The listing builds one solid part. Answer for the finished solid, in the listing's coordinates (mm). Face numbers are marked on the shaded views. A direction names the side the tool comes from. Coordinates: 2 decimals unless noted, no trailing zeros. Loops run counter-clockwise (first coordinate to the right, second up) from the corner with the lowest first, then second, coordinate; pieces in that order, holes last. Notation, with made-up numbers: (39, 22) - (65, 22) arc R18 cw to (65, 35) - close; hole circle Ø8 at (80, 6). An arc over 180 degrees is marked (long way). One line per question, with ' | ' between items.
Autodesk Inventor part; units mm, degrees
ref_plane "YZ Plane" through (0, 0, 0) normal (1, 0, 0) x (0, 1, 0)
ref_plane "XZ Plane" through (0, 0, 0) normal (0, 1, 0) x (-1, 0, 0)
ref_plane "XY Plane" through (0, 0, 0) normal (0, 0, 1) x (1, 0, 0)
sketch "Sketch1" plane through (0, 0, 0) normal (0, 1, 0) x (-1, 0, 0)
  circle A0 centre (0, 0) radius 1.6
  circle A1 centre (0, -62) radius 1.6
  circle A2 centre (25, -62) radius 1.6
  circle A3 centre (12, -31) radius 1.6
  circle A4 centre (12, -31) radius 2.5
  circle A5 centre (0, -62) radius 2.5
  circle A6 centre (25, -62) radius 2.5
  circle A7 centre (0, 0) radius 2.5
  line L0 (30, 5) -> (-5, 5)
  line L1 (-5, 5) -> (-5, -67)
  line L2 (-5, -67) -> (30, -67)
  line L3 (30, -67) -> (30, 5)
  line L4 (33, 8) -> (-8, 8)
  line L5 (-8, 8) -> (-8, -70)
  line L6 (-8, -70) -> (33, -70)
  line L7 (33, -70) -> (33, 8)
  dimension "d0" = 3.2
  dimension "d1" = 3.2
  dimension "d2" = 62
  dimension "d3" = 3.2
  dimension "d4" = 25
  dimension "d5" = 3.2
  dimension "d6" = 31
  dimension "d7" = 12
  dimension "d8" = 5
  dimension "d9" = 5
  dimension "d10" = 5
  dimension "d11" = 5
  dimension "d12" = 5
  dimension "d13" = 5
  dimension "d14" = 5
  dimension "d15" = 5
  dimension "d16" = 3
  dimension "d17" = 3
  dimension "d18" = 3
  dimension "d19" = 3
  dimension "d29" = 0
extrude "Extrusion1" add sketch "Sketch1" along normal blind 12
sketch "Sketch2" plane through (0, 0, 0) normal (0, -1, 0) x (1, 0, 0)
  line L0 (-33, 8) -> (8, 8)
  line L1 (-33, -70) -> (-33, 8)
  line L2 (8, 8) -> (-33, 8)
  line L3 (-33, 8) -> (-33, -70)
  line L4 (-33, -70) -> (8, -70)
  line L5 (8, -70) -> (8, 8)
  point P0 (0, 0)
extrude "Extrusion2" add sketch "Sketch2" along normal blind 4
sketch "Sketch3" plane through (0, 12, 0) normal (0, 1, 0) x (1, 0, 0)
  circle A0 centre (0, 0) radius 1.6
  circle A1 centre (-12, 31) radius 1.6
  circle A2 centre (-25, 62) radius 1.6
  circle A3 centre (0, 62) radius 1.6
extrude "Extrusion3" cut sketch "Sketch3" against normal up to next
sketch "Sketch4" plane through (0, -4, 0) normal (0, -1, 0) x (1, 0, 0)
  circle A0 centre (-25, -62) radius 1.6
  circle A1 centre (-25, -62) radius 4
  circle A2 centre (0, -62) radius 1.6
  circle A3 centre (0, -62) radius 4
  circle A4 centre (-12, -31) radius 1.6
  circle A5 centre (-12, -31) radius 4
  circle A6 centre (0, 0) radius 1.6
  circle A7 centre (0, 0) radius 4
  dimension "d26" = 8
  dimension "d27" = 8
  dimension "d28" = 8
  dimension "d30" = 8
extrude "Extrusion4" cut sketch "Sketch4" against normal blind 2.2
sketch "Sketch6" plane through (0, 12, 0) normal (0, 1, 0) x (1, 0, 0)
  line L0 (-33, 70) -> (-33, -8)
  line L1 (8, 70) -> (-33, 70)
  line L2 (8, -8) -> (8, 70)
  line L3 (-33, -8) -> (8, -8)
  line L4 (-30, -5) -> (-30, 67)
  line L5 (5, -5) -> (-30, -5)
  line L6 (5, 67) -> (5, -5)
  line L7 (-30, 67) -> (5, 67)
  point P0 (0, 0)
extrude "Extrusion5" add sketch "Sketch6" along normal blind 1.6
sketch "Sketch7" plane through (0, 13.6, 0) normal (0, 1, 0) x (1, 0, 0)
  line L0 (-33, 70) -> (-33, -8)
  line L1 (-30, 67) -> (-30, -5)
  line L2 (-33, 20) -> (-30, 20)
  line L3 (-30, 20) -> (-30, 30)
  line L4 (-30, 30) -> (-33, 30)
  line L5 (-33, 30) -> (-33, 20)
  point P0 (0, 0)
  dimension "d35" = 20
  dimension "d36" = 10
extrude "Extrusion6" cut sketch "Sketch7" against normal blind 2
sketch "Sketch8" plane through (8, -4, 8) normal (1, 0, 0) x (0, 0, -1)
  line L0 (78, 17.6) -> (38, 17.6)
  line L1 (0, 0) -> (78, 0)
  line L2 (78, 0) -> (78, 17.6)
  line L3 (78, 17.6) -> (0, 17.6)
  line L4 (0, 17.6) -> (0, 0)
  point P0 (8, 4)
extrude "Extrusion7" add sketch "Sketch8" along normal blind 18
sketch "Sketch9" plane through (0, 13.6, 0) normal (0, 1, 0) x (1, 0, 0)
  line L0 (8, -5) -> (23, -5)
  line L1 (23, -5) -> (23, 67)
  line L2 (23, 67) -> (8, 67)
  line L3 (8, 67) -> (8, -5)
  line L4 (5, 67) -> (5, -5)
  line L5 (26, 70) -> (26, -8)
  line L6 (-33, 70) -> (26, 70)
  point P0 (0, 0)
  dimension "d41" = 3
  dimension "d42" = 3
  dimension "d43" = 3
extrude "Extrusion8" cut sketch "Sketch9" against normal up to surface (13.6 mm away)
properties part number "Housing Base"
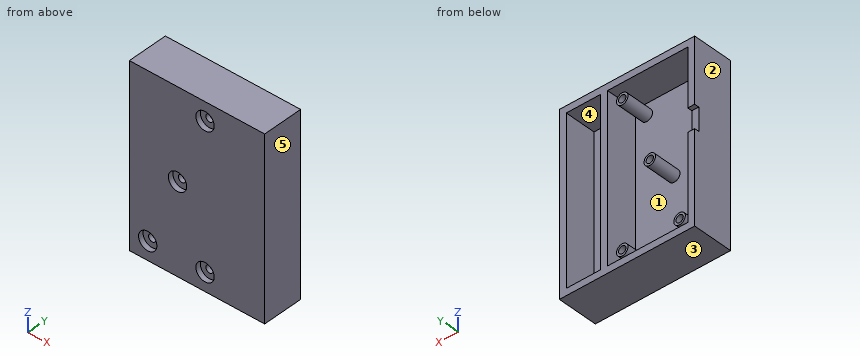
Item 1: Find the intervals of material crossed by line 1 (X direction, y = 7.5, z = -7.5); line 2 (Z direction, x = 0, y = 5.25); line 3 (Z direction, x = -12, y = 5), in increasing order. Write a range as [from, to].
Taken from the geometry:
line 1: x = [-33, -30], [5, 8], [23, 26] | line 2: z = [-70, -67], [-64.5, -63.6], [-60.4, -59.5], [-2.5, -1.6], [1.6, 2.5], [5, 8] | line 3: z = [-70, -67], [-33.5, -32.6], [-29.4, -28.5], [5, 8]
Item 2: Find section D-D, the plane x = -25. Write down the section's boundary in (y, z).
Taken from the geometry:
outline: (-4, -70) - (13.6, -70) - (13.6, -67) - (0, -67) - (0, -64.5) - (12, -64.5) - (12, -63.6) - (-1.8, -63.6) - (-1.8, -66) - (-4, -66) - close; (-4, -58) - (-1.8, -58) - (-1.8, -60.4) - (12, -60.4) - (12, -59.5) - (0, -59.5) - (0, 5) - (13.6, 5) - (13.6, 8) - (-4, 8) - close
Item 3: Find section A-A, the plane z = -31. Write down the section's boundary in (x, y), plus the area to 3 significant figures.
Taken from the geometry:
outline: (-33, -4) - (-16, -4) - (-16, -1.8) - (-13.6, -1.8) - (-13.6, 12) - (-14.5, 12) - (-14.5, 0) - (-30, 0) - (-30, 13.6) - (-33, 13.6) - close; (-10.4, -1.8) - (-8, -1.8) - (-8, -4) - (26, -4) - (26, 13.6) - (23, 13.6) - (23, 0) - (8, 0) - (8, 13.6) - (5, 13.6) - (5, 0) - (-9.5, 0) - (-9.5, 12) - (-10.4, 12) - close | area: 357 mm2
Item 4: Which of the six approach directions +Z, -Z, +X, -X, +Y, -Y give full straight-line access (tool end or side, diameter ignored) to the marked faces 1 and 2?
Taken from the geometry:
face 1: +Y | face 2: +Z, -Z, -X, +Y, -Y
Item 5: Each of these flat-tipped pins is pushed along its axis until it touches: pin 1 Ø2.5 at (x, z) = (-26, -63) entering from +Y; pin 2 Ø4 at (x, z) = (-13, -33) entering from -Y; pin 3 Ø1.9 at (x, z) = (0, -62) entering from -Y; pin 4 Ø6.5 at (x, z) = (0, 0) entering from -Y. Where does it stop, or does it pass through?
Taken from the geometry:
pin 1: stops at y = 12 | pin 2: stops at y = -4 | pin 3: passes through | pin 4: stops at y = -1.8
Item 6: The mould has two halves that part along Z. Classify the marked faces 3, 4 and 5: pulls with the +Z half, pulls with the -Z half, needs draft (parallel to the pull), parting line crosses it, or undercut.
Taken from the geometry:
face 3: pulls with the -Z half | face 4: undercut | face 5: needs draft
Item 7: Find section B-B, the plane x = 0. State how many separate pieces and enclosed holes the cut face has, plus the area to 3 significant figures.
Taken from the geometry:
separate pieces: 3 | enclosed holes: 0 | area: 390 mm2
